from build123d import *

# Parameters (mm, degrees)
F1_DEPTH    = 15.875
F2_R        = 34.925
F3_DEPTH    = 38.1
F3_FACE_R   = 34.925
F3_FACE_R_2 = 18.25625
F5_DEPTH    = 76.2
F6_R        = 4.7625
F7_DEPTH    = 25.4
F8_R        = 4.7625
F9_DEPTH    = 50.8


with BuildPart() as f1:
    # F0 (on Front) → F1 (new body)
    with BuildSketch(Plane.XZ):
        with BuildLine():
            ThreePointArc((0, 73.025), (-51.6364726961, -51.6364726961), (73.025, 0))
            ThreePointArc((73.025, 0), (51.6364726961, 51.6364726961), (0, 73.025))
        make_face()
        with BuildLine():
            ThreePointArc((-31.75, -54.9926131403), (-34.074261314, -46.3183518263), (-25.4, -43.9940905122))
            ThreePointArc((-25.4, -43.9940905122), (-13.1480074912, -49.0690319755), (0, -50.8))
            ThreePointArc((0, -50.8), (6.35, -57.15), (0, -63.5))
            ThreePointArc((0, -63.5), (-16.435009364, -61.3362899694), (-31.75, -54.9926131403))
        make_face(mode=Mode.SUBTRACT)
        with BuildLine():
            ThreePointArc((-31.75, 54.9926131403), (-23.075738686, 52.6683518263), (-25.4, 43.9940905122))
            ThreePointArc((-25.4, 43.9940905122), (-35.9210244843, 35.9210244843), (-43.9940905122, 25.4))
            ThreePointArc((-43.9940905122, 25.4), (-52.6683518263, 23.075738686), (-54.9926131403, 31.75))
            ThreePointArc((-54.9926131403, 31.75), (-44.9012806053, 44.9012806053), (-31.75, 54.9926131403))
        make_face(mode=Mode.SUBTRACT)
        with BuildLine():
            ThreePointArc((18.25625, 0), (-12.909118174, -12.909118174), (0, 18.25625))
            ThreePointArc((0, 18.25625), (9.128125, 15.8103762778), (15.8103762778, 9.128125))
            ThreePointArc((15.8103762778, 9.128125), (17.6341833662, 4.7250651922), (18.25625, 0))
        make_face(mode=Mode.SUBTRACT)
        with BuildLine():
            ThreePointArc((50.8, 0), (49.0690319755, 13.1480074912), (43.9940905122, 25.4))
            ThreePointArc((43.9940905122, 25.4), (46.3183518263, 34.074261314), (54.9926131403, 31.75))
            ThreePointArc((54.9926131403, 31.75), (61.3362899694, 16.435009364), (63.5, 0))
            ThreePointArc((63.5, 0), (57.15, -6.35), (50.8, 0))
        make_face(mode=Mode.SUBTRACT)
    extrude(amount=F1_DEPTH)

    # F2 (on face) → F3 (join)
    with BuildSketch(Plane.XZ.offset(15.875)):
        Circle(F2_R)
        with BuildLine():
            ThreePointArc((-18.25625, 0), (0, 18.25625), (18.25625, 0))
            ThreePointArc((18.25625, 0), (0, -18.25625), (-18.25625, 0))
        make_face(mode=Mode.SUBTRACT)
    extrude(amount=F3_DEPTH)

    # F4 (on Front) + F3_face (on face) → F5 (cut)
    with BuildSketch(Plane.XZ):
        with BuildLine():
            ThreePointArc((-15.7909574359, -9.1616771019), (4.7437852698, -17.6291566836), (18.25625, 0))
            ThreePointArc((18.25625, 0), (18.1000652505, 2.3829187967), (17.6341833662, 4.7250651922))
            Line((17.6341833662, 4.7250651922), (-13.0339616185, -3.4924394899))
            Line((-13.0339616185, -3.4924394899), (-11.8013359162, -8.0926612376))
            Line((-11.8013359162, -8.0926612376), (-15.7909574359, -9.1616771019))
        make_face()
        with BuildLine():
            Line((-13.0339616185, -3.4924394899), (17.6341833662, 4.7250651922))
            ThreePointArc((17.6341833662, 4.7250651922), (-2.363700072, 18.1025850649), (-18.2562088405, 0.0387663935))
            Line((-18.2562088405, 0.0387663935), (-14.2665873208, 1.1077822578))
            Line((-14.2665873208, 1.1077822578), (-13.0339616185, -3.4924394899))
        make_face()
        with BuildLine():
            Line((-21.0017794116, -10.5579126422), (-15.7909574359, -9.1616771019))
            ThreePointArc((-15.7909574359, -9.1616771019), (-16.8591485764, -7.0042682232), (-17.6341833662, -4.7250651922))
            Line((-17.6341833662, -4.7250651922), (-22.2344051139, -5.9576908945))
            Line((-22.2344051139, -5.9576908945), (-21.0017794116, -10.5579126422))
        make_face()
        with BuildLine():
            ThreePointArc((-17.6341833662, -4.7250651922), (-16.8591485764, -7.0042682232), (-15.7909574359, -9.1616771019))
            Line((-15.7909574359, -9.1616771019), (-11.8013359162, -8.0926612376))
            Line((-11.8013359162, -8.0926612376), (-13.0339616185, -3.4924394899))
            Line((-13.0339616185, -3.4924394899), (-17.6341833662, -4.7250651922))
        make_face()
        with BuildLine():
            Line((-14.2665873208, 1.1077822578), (-18.2562088405, 0.0387663935))
            ThreePointArc((-18.2562088405, 0.0387663935), (-18.1025850649, -2.363700072), (-17.6341833662, -4.7250651922))
            Line((-17.6341833662, -4.7250651922), (-13.0339616185, -3.4924394899))
            Line((-13.0339616185, -3.4924394899), (-14.2665873208, 1.1077822578))
        make_face()
        with BuildLine():
            ThreePointArc((-17.6341833662, -4.7250651922), (-18.1025850649, -2.363700072), (-18.2562088405, 0.0387663935))
            Line((-18.2562088405, 0.0387663935), (-18.8668090685, -0.1248434445))
            Line((-18.8668090685, -0.1248434445), (-17.6341833662, -4.7250651922))
        make_face()
        Polygon((-22.2344051139, -5.9576908945), (-17.6341833662, -4.7250651922), (-18.8668090685, -0.1248434445), (-23.4670308162, -1.3574691468), align=None)
    with BuildSketch(Plane.XZ.offset(53.975)):
        Circle(F3_FACE_R)
        Circle(F3_FACE_R_2, mode=Mode.SUBTRACT)
    extrude(amount=F5_DEPTH, mode=Mode.SUBTRACT)

    # F6 (on face) → F7 (cut)
    with BuildSketch(Plane(origin=(-22.2344051139, 0, -5.9576908945), x_dir=(0, 1, 0), z_dir=(0.9659258263, 0, 0.2588190451))):
        with Locations((-34.925, 0)):
            Circle(F6_R)
    extrude(amount=-F7_DEPTH, mode=Mode.SUBTRACT)

    # F8 (on face) → F9 (cut)
    with BuildSketch(Plane(origin=(-1.2326257023, 0, 4.6002217477), x_dir=(0.9659258263, 0, 0.2588190451), z_dir=(0.2588190451, 0, -0.9659258263))):
        with Locations((0, 34.925)):
            Circle(F8_R)
    extrude(amount=-F9_DEPTH, mode=Mode.SUBTRACT)


solid = f1.part
Input: part model. Units: mm. Frame: model coordinates. A direction names the side the tool comes from. Coordinates: 2 decimals unless noted, no trailing zeros. Write each loop counter-clockwise with the first axis right and the second up, starting at its lowest first coordinate (ties: lowest second). Pieces come first, ordered by that corner, then holes. Notation, with made-up numbers: M 62.5,24.25 L 112.5,24.25 A37 ccw 112.5,60.25 Z; hole C 87,58.5 d3. An arc over 180 degrees is marked long. Answer as a JSON object with one key per item and string values. Group by question number.
(1) Mould query, pull axis Z, two halves, no side actions, for faces 3 (the face through (-7.571, -34.658, -34.094)), 4 (the face through (31, -15.875, 17)), 5 (the face through (6.35, -7.83, -57.01)). Classes: pulls with the +Z half, pulls with the -Z half, needs draft (parallel to the pull), parting line crosses it, or undercut.
(2) Set-up query: faces 1 (the face through (61.276, -7.826, 16.66)), 2 (the face through (-7.366, -39.647, 25.095)). Return all of +Z, -Z, +X, -X, +Y, -Y with unobstructed straight access to the full face (end or side cutting, diameter ignored); none if empty.
(3) Section D-D on x = 29. Output: boundary loops of the cut face in (y, z) (3 decimals), plus the area to 3 significant figures.
(4) Section A-A on y = -7. Give the number of separate pieces and of enclosed holes in the cut face, plus the area to 3 significant figures.
(5) Ray query, line 1 along Z through (x, y) = (0, -28) (3 decimals); line 2 along Y through (x, z) = (30, 39.5) (3 decimals); line 3 along Z through (x, y) = (-22, -33). Return the intervals inside material, ascending. Write a range as [from, to].
(6) Section C-C on z = -57.15. Output: boundary loops of the cut face in (x, y) (3 decimals), plus the area to 3 significant figures.
(7) Contact query for flat-ended pins moving along their axis: P1, Ø1.5, axis at x = -30.5, z = 43, coming from the +Y side; P2, Ø4, axis at x = -18, y = -13, coming from the +Z side; P3, Ø10, axis at x = -54.5, y = -7, coming from the +Z side; P4, Ø3, axis at y = -14.5, z = -8, coming from the -X side. Output: stop coordinate, or through.
(8) Section B-B on x = 61.5. Output: boundary loops of the cut face in (y, z) (3 decimals).
Result set:
{
 "1": {"face 3": "parting line crosses it", "face 4": "needs draft", "face 5": "undercut"},
 "2": {"face 1": "+Y, -Y", "face 2": "none"},
 "3": {"outline": "M -53.975,-19.462 L -15.875,-19.462 L -15.875,-67.02 L 0,-67.02 L 0,67.02 L -15.875,67.02 L -15.875,19.462 L -53.975,19.462 Z", "area": "3,610 mm2"},
 "4": {"separate pieces": "1", "enclosed holes": "4", "area": "14,100 mm2"},
 "5": {"line 1": "z = [-34.925, -18.256], [18.256, 34.925]", "line 2": "y = [-15.875, 0]", "line 3": "z = [-27.12, -10.4], [-0.96, 27.12]"},
 "6": {"outline": "M -45.459,-15.875 L -27.679,-15.875 L -27.679,0 L -45.459,0 Z; M 6.35,-15.875 L 45.459,-15.875 L 45.459,0 L 6.35,0 Z", "area": "903 mm2"},
 "7": {"P1": "passes through", "P2": "stops at z = 71.25", "P3": "stops at z = 53.69", "P4": "stops at x = -72.74"},
 "8": {"outline": "M -15.875,-39.375 L 0,-39.375 L 0,-4.626 L -15.875,-4.626 Z; M -15.875,15.811 L 0,15.811 L 0,39.375 L -15.875,39.375 Z"}
}
